Can you work these out from the model? Positions are in its coordinate system, mm. Face numbers are marked on the shaded views. A direction names the side the tool comes from. Give positions to 0.01 mm unless a question says otherwise; leave off trailing zeros. Loops run counter-clockwise (first coordinate to the right, second up) from the corner with the lowest first, then second, coordinate; pieces in that order, holes last. Notation, with made-up numbers: (17.5, 37.25) - (52.5, 37.25) arc R6 ccw to (52.5, 43.25) - close; hole circle Ø9 at (55, 25.25). An arc over 180 degrees is marked (long way). Answer as a JSON object with one key per item and string values.
```python
from build123d import *

# Parameters (mm, degrees)
CROQUIS1_R              = 70
CROQUIS1_R_2            = 28.5
CROQUIS1_R_3            = 6.5
CROQUIS1_R_4            = 5.75
SALIENTE_EXTRUIR1_DEPTH = 19.05
CROQUIS2_R              = 43.95
CROQUIS2_R_2            = 28.5
SALIENTE_EXTRUIR2_DEPTH = 6.35
CROQUIS4_R              = 8.75
CORTAR_EXTRUIR1_DEPTH   = 9.05
MATRIZC1_COUNT          = 4
CROQUIS5_R              = 13
CORTAR_EXTRUIR2_DEPTH   = 19.35
MATRIZC2_COUNT          = 4


with BuildPart() as part:
    # Croquis1 → Saliente-Extruir1 (new body)
    with BuildSketch(Plane.XY):
        Circle(CROQUIS1_R)
        Circle(CROQUIS1_R_2, mode=Mode.SUBTRACT)
        with Locations((35.037141008, 35.037141008)):
            Circle(CROQUIS1_R_3, mode=Mode.SUBTRACT)
        with Locations((35.037141008, -35.037141008)):
            Circle(CROQUIS1_R_3, mode=Mode.SUBTRACT)
        with Locations((-35.037141008, -35.037141008)):
            Circle(CROQUIS1_R_3, mode=Mode.SUBTRACT)
        with Locations((-35.037141008, 35.037141008)):
            Circle(CROQUIS1_R_3, mode=Mode.SUBTRACT)
        with Locations((0, 54)):
            Circle(CROQUIS1_R_4, mode=Mode.SUBTRACT)
        with Locations((54, 0)):
            Circle(CROQUIS1_R_4, mode=Mode.SUBTRACT)
        with Locations((0, -54)):
            Circle(CROQUIS1_R_4, mode=Mode.SUBTRACT)
        with Locations((-54, 0)):
            Circle(CROQUIS1_R_4, mode=Mode.SUBTRACT)
    extrude(amount=-SALIENTE_EXTRUIR1_DEPTH)

    # Croquis2 → Saliente-Extruir2 (add)
    with BuildSketch(Plane.XY):
        Circle(CROQUIS2_R)
        Circle(CROQUIS2_R_2, mode=Mode.SUBTRACT)
    extrude(amount=SALIENTE_EXTRUIR2_DEPTH)

    # Croquis4 → Cortar-Extruir1 (cut)
    with BuildSketch(Plane(origin=(0, 0, -19.05), x_dir=(-1, 0, 0), z_dir=(0, 0, -1))):
        with Locations((0, 54)):
            Circle(CROQUIS4_R)
    cortar_extruir1 = extrude(amount=-CORTAR_EXTRUIR1_DEPTH, mode=Mode.SUBTRACT)

    # MatrizC1: Cortar-Extruir1 ×4 about axis
    matrizc1_axis = Axis((0, 0, 0), (0, 0, 1))
    for i in range(1, MATRIZC1_COUNT):
        add(cortar_extruir1.rotate(matrizc1_axis, i * 360 / MATRIZC1_COUNT), mode=Mode.SUBTRACT)

    # Croquis5 → Cortar-Extruir2 (cut)
    with BuildSketch(Plane.XY.offset(6.35)):
        with Locations((-35.037141008, 35.037141008)):
            Circle(CROQUIS5_R)
    cortar_extruir2 = extrude(amount=-CORTAR_EXTRUIR2_DEPTH, mode=Mode.SUBTRACT)

    # MatrizC2: Cortar-Extruir2 ×4 about axis
    matrizc2_axis = Axis((0, 0, 0), (0, 0, 1))
    for i in range(1, MATRIZC2_COUNT):
        add(cortar_extruir2.rotate(matrizc2_axis, i * 360 / MATRIZC2_COUNT), mode=Mode.SUBTRACT)


solid = part.part
```
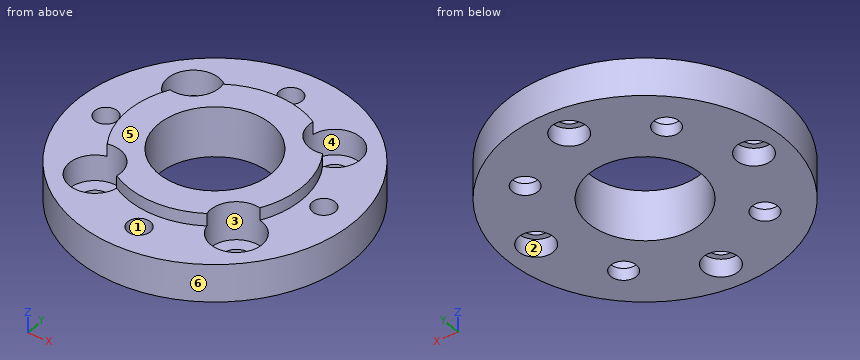
1) Imagine slicing it at A-A on y = 0. Write out the boundary of the cut face in (x, z), and give its area (3 significant figures).
Check sheet entries:
{"outline": "(-70, -19.05) - (-62.75, -19.05) - (-62.75, -10) - (-59.75, -10) - (-59.75, 0) - (-70, 0) - close; (-48.25, -10) - (-45.25, -10) - (-45.25, -19.05) - (-28.5, -19.05) - (-28.5, 6.35) - (-43.95, 6.35) - (-43.95, 0) - (-48.25, 0) - close; (28.5, -19.05) - (45.25, -19.05) - (45.25, -10) - (48.25, -10) - (48.25, 0) - (43.95, 0) - (43.95, 6.35) - (28.5, 6.35) - close; (59.75, -10) - (62.75, -10) - (62.75, -19.05) - (70, -19.05) - (70, 0) - (59.75, 0) - close", "area": "1,230 mm2"}
2) I need wall thicknesses on L1, parallel to Y at x = 0, z = -3.25; L2, parallel to X at y = -7.5, z = -17.25; L3, parallel to Y at x = 42, z = -5.75. Which ranges of each line are inside material? Lowest first, please.
Check sheet entries:
{"L1": "-70 to -59.75, -48.25 to -28.5, 28.5 to 48.25, 59.75 to 70", "L2": "-69.6 to -58.51, -49.49 to -27.5, 27.5 to 49.49, 58.51 to 69.6", "L3": "-56 to -46.02, -24.06 to 24.06, 46.02 to 56"}
3) Imagine slicing it at C-C on x = -54. Write out the boundary of the cut face in (y, z).
Check sheet entries:
{"outline": "(-44.54, -19.05) - (-8.75, -19.05) - (-8.75, -10) - (-5.75, -10) - (-5.75, 0) - (-44.54, 0) - close; (5.75, -10) - (8.75, -10) - (8.75, -19.05) - (44.54, -19.05) - (44.54, 0) - (5.75, 0) - close"}
4) Which directions (+Z, -Z, +X, -X, +Y, -Y) give clear straight access to the entire face, cutting with the end or side of a thin tool? Please do the marked faces 1, 2 and 3.
Check sheet entries:
{"face 1": "+Z, -Z", "face 2": "-Z", "face 3": "+Z"}
5) If we mould it in two halves opening along X, with no side actions, what happens to the marked faces 4, 5 and 6? For each: released by +X, released by -X, zero draft, split by the parting line, or undercut.
Check sheet entries:
{"face 4": "undercut", "face 5": "zero draft", "face 6": "split by the parting line"}
6) I'm going to push flat-ended pins straight in: P1, Ø19, axis at x = 0.5, y = -52.5, coming from the -Z side; P2, Ø1, axis at x = -26, z = -4.5, coming from the -Y side; P3, Ø15, axis at x = 54, y = 0, coming from the +Z side; P4, Ø1.5, axis at x = -27, z = -12.5, coming from the +Y side. Where does each tip first touch, or does it pass through?
Check sheet entries:
{"P1": "z = -19.05", "P2": "y = -65.19", "P3": "z = 0", "P4": "y = 64.89"}
7) Imagine slicing it at D-D on z = -16.5. Give the number of separate pieces and of enclosed holes in the cut face, and give its area (3 significant figures).
Check sheet entries:
{"separate pieces": "1", "enclosed holes": "9", "area": "11,300 mm2"}
